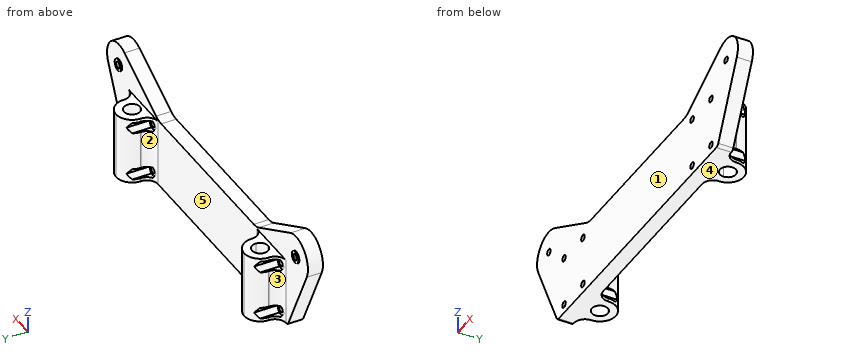
from build123d import *

# Parameters (mm, degrees)
SKETCH1_W               = 30
SKETCH1_H               = 34
BOSS_EXTRUDE1_DEPTH     = 7.5
BOSS_EXTRUDE2_DEPTH     = 34
CUT_EXTRUDE2_DEPTH      = 34
CUT_EXTRUDE2_DEPTH_BACK = 34
SKETCH5_R               = 1.6
CUT_EXTRUDE3_DEPTH      = 34
SKETCH6_R               = 1.6
BOSS_EXTRUDE3_DEPTH     = 7.5
SKETCH7_R               = 3
SKETCH7_R_2             = 1.6
BOSS_EXTRUDE4_DEPTH     = 0.5
FILLET1_R               = 2
BOSS_EXTRUDE5_START     = -7.5
BOSS_EXTRUDE5_DEPTH     = 7.5
FILLET2_R               = 10


with BuildPart() as part:
    # Sketch1 → Boss-Extrude1 (new body)
    with BuildSketch(Plane(origin=(0, 0, 0), x_dir=(1, 0, 0), z_dir=(0, 1, 0))):
        Rectangle(SKETCH1_W, SKETCH1_H)
    extrude(amount=BOSS_EXTRUDE1_DEPTH)

    # Sketch2 → Boss-Extrude2 (add)
    with BuildSketch(Plane.XY.offset(17)):
        with BuildLine():
            ThreePointArc((8, 13.207420741), (5.656854249, 18.86427499), (0, 21.207420741))
            Line((0, 21.207420741), (0, 17.207420741))
            ThreePointArc((0, 17.207420741), (2.828427125, 16.035847865), (4, 13.207420741))
            ThreePointArc((4, 13.207420741), (2.828427125, 10.378993616), (0, 9.207420741))
            Line((0, 9.207420741), (0, 7.5))
            Line((0, 7.5), (5.60583165, 7.5))
            ThreePointArc((5.60583165, 7.5), (7.377216725, 10.112800667), (8, 13.207420741))
        make_face()
        with BuildLine():
            ThreePointArc((0, 21.207420741), (-5.656854249, 18.86427499), (-8, 13.207420741))
            ThreePointArc((-8, 13.207420741), (-7.377216725, 10.112800667), (-5.60583165, 7.5))
            Line((-5.60583165, 7.5), (0, 7.5))
            Line((0, 7.5), (0, 9.207420741))
            ThreePointArc((0, 9.207420741), (-4, 13.207420741), (0, 17.207420741))
            Line((0, 17.207420741), (0, 21.207420741))
        make_face()
        with BuildLine():
            Line((8, 13), (8, 13.207420741))
            ThreePointArc((8, 13.207420741), (7.377216725, 10.112800667), (5.60583165, 7.5))
            Line((5.60583165, 7.5), (13.5, 7.5))
            ThreePointArc((13.5, 7.5), (9.610912703, 9.110912703), (8, 13))
        make_face()
        with BuildLine():
            ThreePointArc((-5.60583165, 7.5), (-7.377216725, 10.112800667), (-8, 13.207420741))
            Line((-8, 13.207420741), (-8, 13))
            ThreePointArc((-8, 13), (-9.610912703, 9.110912703), (-13.5, 7.5))
            Line((-13.5, 7.5), (-5.60583165, 7.5))
        make_face()
    extrude(amount=-BOSS_EXTRUDE2_DEPTH)

    # Sketch5 → Cut-Extrude2 (cut, two sides: drawn at the far end of the back side and taken through both)
    with BuildSketch(Plane(origin=(0, 7.5, 0), x_dir=(1, 0, 0), z_dir=(0, 1, 0)).offset(-CUT_EXTRUDE2_DEPTH_BACK)):
        with Locations(Location((-8.75, 12.5, 0), (0, 0, 62.046813117))):
            Circle(SKETCH5_R)
        with Locations(Location((8.75, 12.5, 0), (0, 0, 117.953186883))):
            Circle(SKETCH5_R)
        with Locations(Location((-8.75, -12.5, 0), (0, 0, 62.046813117))):
            Circle(SKETCH5_R)
        with Locations(Location((8.75, -12.5, 0), (0, 0, 117.953186883))):
            Circle(SKETCH5_R)
    extrude(amount=CUT_EXTRUDE2_DEPTH + CUT_EXTRUDE2_DEPTH_BACK, mode=Mode.SUBTRACT)

    # Sketch5<3> → Cut-Extrude3 (cut)
    with BuildSketch(Plane(origin=(0, 7.5, 0), x_dir=(1, 0, 0), z_dir=(0, 1, 0))):
        Polygon((7.133419246, -9.7), (10.366580754, -9.7), (11.983161507, -12.5), (10.366580754, -15.3), (7.133419246, -15.3), (5.516838493, -12.5), align=None)
        Polygon((-12.098631561, 12.5), (-10.424315781, 9.6), (-7.075684219, 9.6), (-5.401368439, 12.5), (-7.075684219, 15.4), (-10.424315781, 15.4), align=None)
        Polygon((5.516838493, 12.5), (7.133419246, 9.7), (10.366580754, 9.7), (11.983161507, 12.5), (10.366580754, 15.3), (7.133419246, 15.3), align=None)
        Polygon((-7.075684219, -9.6), (-5.401368439, -12.5), (-7.075684219, -15.4), (-10.424315781, -15.4), (-12.098631561, -12.5), (-10.424315781, -9.6), align=None)
    extrude(amount=CUT_EXTRUDE3_DEPTH, mode=Mode.SUBTRACT)

    # Sketch6 → Boss-Extrude3 (add)
    with BuildSketch(Plane.XZ):
        with BuildLine():
            Line((-32.702629656, 20.034210881), (-15, -17))
            Line((-15, -17), (-15, 17))
            Line((-15, 17), (15, 17))
            Line((15, 17), (-17.579374925, 34.472115072))
            ThreePointArc((-17.579374925, 34.472115072), (-30.37397765, 32.734541598), (-32.702629656, 20.034210881))
        make_face()
        with Locations(Location((-22.778174593, 24.778174593, 0), (0, 0, 270))):
            Circle(SKETCH6_R, mode=Mode.SUBTRACT)
    extrude(amount=-BOSS_EXTRUDE3_DEPTH)

    # Sketch7 → Boss-Extrude4 (add)
    with BuildSketch(Plane(origin=(0, 7.5, 0), x_dir=(1, 0, 0), z_dir=(0, 1, 0))):
        with Locations(Location((-22.778174593, -24.778174593, 0), (0, 0, 270))):
            Circle(SKETCH7_R)
        with Locations(Location((-22.778174593, -24.778174593, 0), (0, 0, 90))):
            Circle(SKETCH7_R_2, mode=Mode.SUBTRACT)
    extrude(amount=BOSS_EXTRUDE4_DEPTH)

    # Fillet1
    fillet1_edges = [part.edges().sort_by_distance(p)[0] for p in [
        (-15, 3.75, -17),
        (15, 3.75, -17),
        (15, 3.75, 17),
    ]]
    fillet(fillet1_edges, radius=FILLET1_R)

    # Sketch8 → Boss-Extrude5 (add)
    with BuildSketch(Plane.XZ.offset(BOSS_EXTRUDE5_START)):
        with BuildLine():
            ThreePointArc((15, -15), (14.414213562, -16.414213562), (13, -17))
            Line((13, -17), (59.4, -17))
            Line((59.4, -17), (59.4, 17.565663176))
            Line((59.4, 17.565663176), (13.945236303, 17.565663176))
            ThreePointArc((13.945236303, 17.565663176), (14.716169078, 16.830145435), (15, 15.803128543))
            Line((15, 15.803128543), (15, -15))
        make_face()
    extrude(amount=BOSS_EXTRUDE5_DEPTH)

    # Mirror3: part across plane


with BuildPart() as part_1:
    add(part.part)
    add(part.part.mirror(Plane(origin=(59.4, 7.5, 0), x_dir=(0, 0, 1), z_dir=(-1, 0, 0))))

    # Fillet2
    fillet2_edges = [part_1.edges().sort_by_distance(p)[0] for p in [
        (13.945236303, 3.75, 17.565663176),
        (104.854763697, 3.75, 17.565663176),
    ]]
    fillet(fillet2_edges, radius=FILLET2_R)


solid = part_1.part
Model file for the job. Use its own axes, mm. Face numbers are marked on the shaded views. A direction names the side the tool comes from. Round coordinates to 2 decimals unless told otherwise and drop trailing zeros. Loops run counter-clockwise (first coordinate to the right, second up) from the corner with the lowest first, then second, coordinate; pieces in that order, holes last. Notation, with made-up numbers: (26, 78.5) - (30, 78.5) arc R25 cw to (30, 92.5) - close; hole circle Ø10 at (1, 86). An arc over 180 degrees is marked (long way). Write each question's results on one line, items separated by ' | '.
(1) Pin check, flat tips, straight feed: pin 1 (1.5 mm diameter, centred on y = 17, z = -10, fed in from +X); pin 2 (4 mm diameter, centred on x = 79.5, z = 16, fed in from +Y); pin 3 (2 mm diameter, centred on x = 73, y = 4, fed in from +Z); pin 4 (1.6 mm diameter, centred on x = 109.5, y = 12.5, fed in from +Z). Stop position of each tip, or through.
Answer below:
pin 1: stops at x = 126.15 | pin 2: stops at y = 7.5 | pin 3: stops at z = 17.57 | pin 4: passes through
(2) Wall check: L1, parallel to Z at x = 127.5, y = 8; L2, parallel to Z at x = -8.75, y = 2.25; L3, parallel to X at y = 11.25, z = -5. Give the ranges that are in metal, low to high.
Answer below:
L1: z = -17 to -15.4, -9.6 to 9.6, 15.4 to 17 | L2: z = -17 to -14.1, -10.9 to 10.9, 14.1 to 29.74 | L3: x = -8.29 to -3.49, 3.49 to 8.29, 110.51 to 115.31, 122.29 to 127.09
(3) Saw through at A-A, the plane z = -4. List the corners of the cut face in (x, y).
Answer below:
outline: (-21.21, 0) - (140.01, 0) - (140.01, 7.5) - (132.3, 7.5) arc R5.5 cw to (126.8, 13) - (126.8, 13.21) arc R8 ccw to (110.8, 13.21) - (110.8, 13) arc R5.5 cw to (105.3, 7.5) - (13.5, 7.5) arc R5.5 cw to (8, 13) - (8, 13.21) arc R8 ccw to (-8, 13.21) - (-8, 13) arc R5.5 cw to (-13.5, 7.5) - (-21.21, 7.5) - close; hole circle Ø8 at (0, 13.21); hole circle Ø8 at (118.8, 13.21)
(4) Saw through at B-B, the plane y = 5.75. Count the separate pieces of the cut face and the enclosed holes in it, then the cut area to 3 significant figures.
Answer below:
separate pieces: 1 | enclosed holes: 10 | area: 6,690 mm^2
(5) Mould opens along X. For the marked faces 3, 4 and 5 say: released by +X, released by -X, zero draft, split by the parting line, or undercut.
Answer below:
face 3: released by -X | face 4: zero draft | face 5: undercut
(6) 3-axis set-ups, long thin cutter, end or side, ignore diameter. For the marked faces 1 and 2: which of +Z, -Z, +X, -X, +Y, -Y reach the whole face in a straight line?
Answer below:
face 1: +Z, -Z, +X, -X, -Y | face 2: +Z, -Z, +Y
(7) Saw through at C-C, the plane x = 54.5. List the corners of the cut face in (y, z).
Answer below:
outline: (0, -17) - (7.5, -17) - (7.5, 17.57) - (0, 17.57) - close
